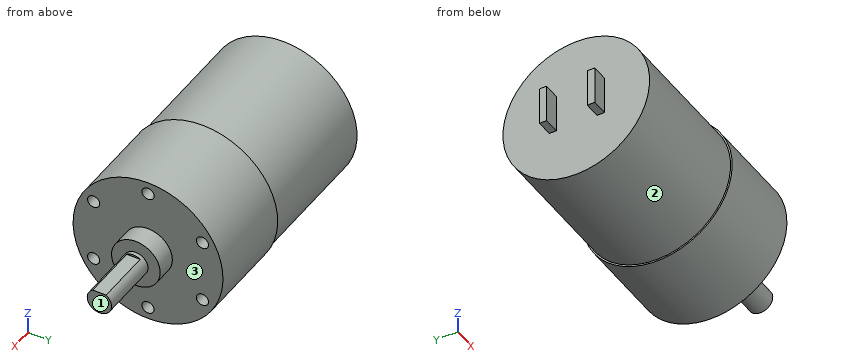
```python
from build123d import *

# Parameters (mm, degrees)
SKETCH1_R               = 18.5
BOSS_EXTRUDE1_DEPTH     = 22.5
SKETCH2_R               = 6
BOSS_EXTRUDE2_DEPTH     = 5
SKETCH3_R               = 3
BOSS_EXTRUDE3_DEPTH     = 15
CUT_EXTRUDE1_DEPTH      = 50.907414279
CUT_EXTRUDE1_DEPTH_BACK = 14
SKETCH5_R               = 18.1
BOSS_EXTRUDE4_DEPTH     = 33.3
SKETCH6_W               = 1.743362505
SKETCH6_H               = 9.378087958
SKETCH6_W_2             = 1.863594402
BOSS_EXTRUDE5_DEPTH     = 4
SKETCH7_R               = 1.5
CUT_EXTRUDE2_DEPTH      = 5


with BuildPart() as part:
    # Sketch1 → Boss-Extrude1 (new body)
    with BuildSketch(Plane.YZ):
        with Locations(Location((0, 0, 0), (0, 0, 90))):
            Circle(SKETCH1_R)
    extrude(amount=BOSS_EXTRUDE1_DEPTH)

    # Sketch2 → Boss-Extrude2 (add)
    with BuildSketch(Plane.YZ.offset(22.5)):
        with Locations(Location((0, 0, 0), (0, 0, 270))):
            Circle(SKETCH2_R)
    extrude(amount=BOSS_EXTRUDE2_DEPTH)

    # Sketch3 → Boss-Extrude3 (add)
    with BuildSketch(Plane.YZ.offset(27.5)):
        with Locations(Location((0, 0, 0), (0, 0, 270))):
            Circle(SKETCH3_R)
    extrude(amount=BOSS_EXTRUDE3_DEPTH)

    # Sketch4 → Cut-Extrude1 (cut, two sides: drawn at the far end of the back side and taken through both)
    with BuildSketch(Plane.YZ.offset(42.5).offset(-CUT_EXTRUDE1_DEPTH_BACK)):
        Polygon((-69.877125802, 2.5), (-1.658312395, 2.5), (1.658312395, 2.5), (69.877125802, 2.5), (69.877125802, 138.937626813), (-69.877125802, 138.937626813), align=None)
    extrude(amount=CUT_EXTRUDE1_DEPTH + CUT_EXTRUDE1_DEPTH_BACK, mode=Mode.SUBTRACT)

    # Sketch5 → Boss-Extrude4 (add)
    with BuildSketch(Plane(origin=(0, 0, 0), x_dir=(0, -1, 0), z_dir=(-1, 0, 0))):
        with Locations(Location((0, 0, 0), (0, 0, 90))):
            Circle(SKETCH5_R)
    extrude(amount=BOSS_EXTRUDE4_DEPTH)

    # Sketch6 → Boss-Extrude5 (add)
    with BuildSketch(Plane(origin=(-33.3, 0, 0), x_dir=(0, -1, 0), z_dir=(-1, 0, 0))):
        with Locations((-5.801189026, 0.510985562)):
            Rectangle(SKETCH6_W, SKETCH6_H)
        with Locations((6.041652819, 0.510985562)):
            Rectangle(SKETCH6_W_2, SKETCH6_H)
    extrude(amount=BOSS_EXTRUDE5_DEPTH)

    # Sketch7 → Cut-Extrude2 (cut)
    with BuildSketch(Plane.YZ.offset(22.5)):
        with Locations(Location((0, 15.5, 0), (0, 0, 270))):
            Circle(SKETCH7_R)
        with Locations(Location((13.423393759, 7.75, 0), (0, 0, 270))):
            Circle(SKETCH7_R)
        with Locations(Location((13.423393759, -7.75, 0), (0, 0, 270))):
            Circle(SKETCH7_R)
        with Locations(Location((0, -15.5, 0), (0, 0, 270))):
            Circle(SKETCH7_R)
        with Locations(Location((-13.423393759, -7.75, 0), (0, 0, 270))):
            Circle(SKETCH7_R)
        with Locations(Location((-13.423393759, 7.75, 0), (0, 0, 270))):
            Circle(SKETCH7_R)
    extrude(amount=-CUT_EXTRUDE2_DEPTH, mode=Mode.SUBTRACT)


solid = part.part
```
Can you work these out from the model? Positions are in its coordinate system, mm. Face numbers are marked on the shaded views. A direction names the side the tool comes from. Give positions to 0.01 mm unless a question says otherwise; leave off trailing zeros. Loops run counter-clockwise (first coordinate to the right, second up) from the corner with the lowest first, then second, coordinate; pieces in that order, holes last. Notation, with made-up numbers: M 10,39.5 L 23,39.5 A16 ccw 23,58.5 Z; hole C 75.5,29.25 d5. An arc over 180 degrees is marked long. Answer in a Markdown table with one row per item.
1. Suppose I cut it at C-C on x = 30. Write out the boundary of the cut face in (y, z).
Taken from the geometry:
| item | result |
|---|---|
| outline | M -1.66,2.5 A3 ccw long 1.66,2.5 Z |
2. Suppose I cut it at D-D on y = 8. Write out the boundary of the cut face in (x, z), plus the area to 3 significant figures.
Taken from the geometry:
| item | result |
|---|---|
| outline | M -33.3,-16.24 L 0,-16.24 L 0,-16.68 L 22.5,-16.68 L 22.5,16.68 L 0,16.68 L 0,16.24 L -33.3,16.24 Z |
| area | 1,830 mm² |
3. If I drill on line 1 along Y through (x, z) = (19.95, 7.75); line 2 along X through (y, z) = (-6.5, 10.5); line 3 along X through (y, z) = (-4.5, -0.5), over which ranges is the centre line in solid material (lowest first)?
Taken from the geometry:
| item | result |
|---|---|
| line 1 | y = -16.8 to -14.92, -11.92 to 11.92, 14.92 to 16.8 |
| line 2 | x = -33.3 to 22.5 |
| line 3 | x = -33.3 to 27.5 |
4. For pin 1 Ø5 at (x, y) = (-23.5, 8) entering from -Z; pin 2 Ø1.4 at (x, y) = (-35.5, 6) entering from -Z; pin 3 Ø2.5 at (y, z) = (14, -8) entering from +X; pin 4 Ø3.5 at (y, z) = (-2, -3) entering from +X, each with a flat end and sliding along its axis, tell me the tip position at first contact or that it passes through.
Taken from the geometry:
| item | result |
|---|---|
| pin 1 | stops at z = -17.24 |
| pin 2 | stops at z = -4.18 |
| pin 3 | stops at x = 22.5 |
| pin 4 | stops at x = 42.5 |
5. Suppose I cut it at A-A on y = 0. Write out the boundary of the cut face in (x, z).
Taken from the geometry:
| item | result |
|---|---|
| outline | M -33.3,-18.1 L 0,-18.1 L 0,-18.5 L 22.5,-18.5 L 22.5,-17 L 17.5,-17 L 17.5,-14 L 22.5,-14 L 22.5,-6 L 27.5,-6 L 27.5,-3 L 42.5,-3 L 42.5,2.5 L 28.5,2.5 L 28.5,3 L 27.5,3 L 27.5,6 L 22.5,6 L 22.5,14 L 17.5,14 L 17.5,17 L 22.5,17 L 22.5,18.5 L 0,18.5 L 0,18.1 L -33.3,18.1 Z |
6. Which directions (+Z, -Z, +X, -X, +Y, -Y) give clear straight access to the entire face, cutting with the end or side of a thin tool? Please do the marked faces 1, 2 and 3.
Taken from the geometry:
| item | result |
|---|---|
| face 1 | +Z, -Z, +X, +Y, -Y |
| face 2 | -X |
| face 3 | +X |
7. Suppose I cut it at B-B on z = 0. Write out the boundary of the cut face in (x, y).
Taken from the geometry:
| item | result |
|---|---|
| outline | M -37.3,-6.97 L -33.3,-6.97 L -33.3,-18.1 L 0,-18.1 L 0,-18.5 L 22.5,-18.5 L 22.5,-6 L 27.5,-6 L 27.5,-3 L 42.5,-3 L 42.5,3 L 27.5,3 L 27.5,6 L 22.5,6 L 22.5,18.5 L 0,18.5 L 0,18.1 L -33.3,18.1 L -33.3,6.67 L -37.3,6.67 L -37.3,4.93 L -33.3,4.93 L -33.3,-5.11 L -37.3,-5.11 Z |
